```python
from build123d import *

# Parameters (mm, degrees)
F1_DEPTH = 6.35
F3_D     = 4.4958
F4_R     = 11.1125
F5_DEPTH = 9.525


with BuildPart() as f1:
    # F0 (on Front) → F1 (new body)
    with BuildSketch(Plane.XZ):
        with BuildLine():
            Line((18.2969275085, 15.24), (-18.2969275085, 15.24))
            ThreePointArc((-18.2969275085, 15.24), (0, -23.8125), (18.2969275085, 15.24))
        make_face()
    extrude(amount=F1_DEPTH)

    # F3 (through all)
    with Locations(Plane.XZ.offset(6.35)):
        with Locations((-9.525, -15.7602855304), (-15.7602855304, 9.525), (15.7602855304, 9.525), (9.525, -15.7602855304)):
            Hole(F3_D / 2)

    # F4 (on face) → F5 (join)
    with BuildSketch(Plane.XZ.offset(6.35)):
        Circle(F4_R)
    extrude(amount=F5_DEPTH)


solid = f1.part
```
For this review, take the finished solid that the model builds, in its own axes (mm). A direction names the side the tool comes from. Give positions to 0.01 mm unless a question says otherwise; leave off trailing zeros. Write each loop counter-clockwise with the first axis right and the second up, starting at its lowest first coordinate (ties: lowest second). Pieces come first, ordered by that corner, then holes. Notation, with made-up numbers: M 79.25,-12.75 L 132.25,-12.75 A7 cw 132.25,-2.75 Z; hole C 19.25,57.25 d3. An arc over 180 degrees is marked long. One line per item, written item: value.
1) For faces 1 (the flat face through (0, -3, 15.24)), 2 (the flat face through (0, -6.35, -13)), list the 3-axis set-ups (+Z, -Z, +X, -X, +Y, -Y) from which the entire face can be reached by the end or side of a thin tool; tool diameter is ignored.
Results are:
face 1: +Z, +X, -X, +Y, -Y
face 2: -Y
2) For line 1 (X direction, y = -6, z = -16); line 2 (X direction, y = -5, z = -14); line 3 (Y direction, x = -19, z = -14), list the stretches that pass through material, from the lowest coordinate up. Write a range as from..to.
Results are:
line 1: x = -17.64..-11.76, -7.29..7.29, 11.76..17.64
line 2: x = -19.26..-10.92, -8.13..8.13, 10.92..19.26
line 3: y = -6.35..0
3) Take a section at A-A, the plane x = -17. Write out the cut boundary in (y, z), then the cut area to 3 significant figures.
Results are:
outline: M -6.35,-16.67 L 0,-16.67 L 0,7.65 L -6.35,7.65 Z; M -6.35,11.4 L 0,11.4 L 0,15.24 L -6.35,15.24 Z
area: 179 mm²
4) The part is to be moulded in two halves that separate along X. For faces 3 (the flat face through (0, -15.875, 0)), 4 (the cylindrical face through (17.544, -3.131, 8.157)), 5 (the cylindrical face through (-0.8, -3.1, -23.8)), say which applies: +X half, -X half, draft (parallel to the pull), parting line (faces both ways), or undercut.
Results are:
face 3: draft
face 4: undercut
face 5: parting line
5) For P1, Ø3, axis at x = -5, z = -13, coming from the -Y side; P2, Ø3, axis at x = 7, y = -4.5, coming from the -Z side, all flat-tipped, find the tip position at first contact; note any pin that passes through.
Results are:
P1: stops at y = -6.35
P2: stops at z = -23.17
6) Take a section at D-D, the plane y = -13.75. Write out the cut boundary in (x, z) (1 decimal).
Results are:
outline: C 0,0 d22.2
